```python
from build123d import *

# Parameters (mm, degrees)
SKETCH1_W           = 101
SKETCH1_H           = 59.932047928
SKETCH1_R           = 11
SKETCH1_R_2         = 10
BOSS_EXTRUDE1_DEPTH = 50
SKETCH3_R           = 17
CUT_EXTRUDE1_DEPTH  = 10
SKETCH4_R           = 20
CUT_EXTRUDE2_DEPTH  = 39


with BuildPart() as part:
    # Sketch1 → Boss-Extrude1 (new body)
    with BuildSketch(Plane(origin=(0, 0, 0), x_dir=(1, 0, 0), z_dir=(0, 1, 0))):
        Rectangle(SKETCH1_W, SKETCH1_H)
        with Locations(Location((-20.5, 0, 0), (0, 0, 270))):
            Circle(SKETCH1_R, mode=Mode.SUBTRACT)
        with Locations(Location((20.5, 0, 0), (0, 0, 270))):
            Circle(SKETCH1_R_2, mode=Mode.SUBTRACT)
    extrude(amount=BOSS_EXTRUDE1_DEPTH)

    # Sketch3 → Cut-Extrude1 (cut)
    with BuildSketch(Plane.XZ):
        with Locations(Location((-20.5, 0, 0), (0, 0, 270))):
            Circle(SKETCH3_R)
    extrude(amount=-CUT_EXTRUDE1_DEPTH, mode=Mode.SUBTRACT)

    # Sketch4 → Cut-Extrude2 (cut)
    with BuildSketch(Plane(origin=(0, 50, 0), x_dir=(1, 0, 0), z_dir=(0, 1, 0))):
        with Locations(Location((-20.5, 0, 0), (0, 0, 270))):
            Circle(SKETCH4_R)
    extrude(amount=-CUT_EXTRUDE2_DEPTH, mode=Mode.SUBTRACT)


solid = part.part
```
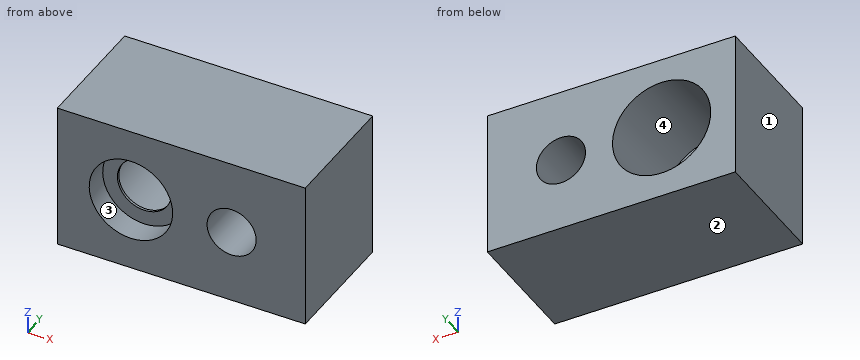
Work out the finished part from the listing and answer in its coordinate system (mm). Face numbers are marked on the shaded views. Round coordinates to 2 decimals unless told otherwise and drop trailing zeros. Write each loop counter-clockwise with the first axis right and the second up, starting at its lowest first coordinate (ties: lowest second). Pieces come first, ordered by that corner, then holes. Notation, with made-up numbers: (-20, 17) -> (20, 17) arc R25 ccw to (20, 38) -> close; hole circle Ø3 at (-19.5, -39). An arc over 180 degrees is marked (long way). Write each question's results on one line, items separated by ' | '.
Q1. Section A-A, the plane x = 20.5 is taken. Write down the section's boundary in (y, z), then the cut area to 3 significant figures.
Data:
outline: (0, -29.97) -> (50, -29.97) -> (50, -10) -> (0, -10) -> close; (0, 10) -> (50, 10) -> (50, 29.97) -> (0, 29.97) -> close | area: 2,000 mm^2
Q2. A flat-ended cylindrical pin translates along its axis: P1, Ø10, axis at x = 5, z = 2.5, coming from the -Y side. Find the tip coordinate at first contact, or state that the pin passes through.
Data:
P1: y = 0
Q3. Section D-D, the plane x = -20.5 is taken. Write down the section's boundary in (y, z), then the cut area to 3 significant figures.
Data:
outline: (0, -29.97) -> (50, -29.97) -> (50, -20) -> (11, -20) -> (11, -11) -> (10, -11) -> (10, -17) -> (0, -17) -> close; (0, 17) -> (10, 17) -> (10, 11) -> (11, 11) -> (11, 20) -> (50, 20) -> (50, 29.97) -> (0, 29.97) -> close | area: 1,070 mm^2
Q4. Section C-C, the plane y = 39 is taken. Write down the section's boundary in (x, z), then the cut area to 3 significant figures.
Data:
outline: (-50.5, -29.97) -> (50.5, -29.97) -> (50.5, 29.97) -> (-50.5, 29.97) -> close; hole circle Ø40 at (-20.5, 0); hole circle Ø20 at (20.5, 0) | area: 4,480 mm^2
Q5. Section B-B, the plane z = -5 is taken. Write down the section's boundary in (x, y).
Data:
outline: (-50.5, 0) -> (-36.75, 0) -> (-36.75, 10) -> (-30.3, 10) -> (-30.3, 11) -> (-39.86, 11) -> (-39.86, 50) -> (-50.5, 50) -> close; (-10.7, 10) -> (-4.25, 10) -> (-4.25, 0) -> (11.84, 0) -> (11.84, 50) -> (-1.14, 50) -> (-1.14, 11) -> (-10.7, 11) -> close; (29.16, 0) -> (50.5, 0) -> (50.5, 50) -> (29.16, 50) -> close
Q6. Determine the mould class of the marked faces 1, 2, 3 and 4 for opening direction X: released by +X, released by -X, zero draft, split by the parting line, or undercut.
Data:
face 1: released by -X | face 2: zero draft | face 3: undercut | face 4: undercut
Q7. Straight lines are drawn through the part: line 1 along X through (y, z) = (5, 0); line 2 along X through (y, z) = (26.5, 0); line 3 along Z through (x, y) = (-21, 31). For each, find the intervals that lie inside material, in ascending order. Write a range as [from, to].
Data:
line 1: [-50.5, -37.5], [-3.5, 10.5], [30.5, 50.5] | line 2: [-50.5, -40.5], [-0.5, 10.5], [30.5, 50.5] | line 3: [-29.97, -19.99], [19.99, 29.97]
